Build history of the part. All positions in model axes, mm. A direction names the side the tool comes from. Round coordinates to 2 decimals unless told otherwise and drop trailing zeros. Write each loop counter-clockwise with the first axis right and the second up, starting at its lowest first coordinate (ties: lowest second). Pieces come first, ordered by that corner, then holes.
Item 1: Wall check: probe 1 along Y at (x, z) = (-3, 3.65); probe 2 along X at (y, z) = (5, 0.25); probe 3 along Y at (x, z) = (-14, 3.25). Give the ranges that are in metal, low to high.
Item 2: Band-saw the part on B-B, the plane y = 4.5. Write the cut outline in (x, z), then the cut area to 4 significant figures.
Item 3: Band-saw the part on A-A, the plane x = 3. Write the cut outline in (y, z).
Item 4: 3-axis set-ups, long thin cutter, end or side, ignore diameter. For faces 5 (the flat face through (-16, -6.3, 2)), 6 (the flat face through (-6.2, -9, 2)), 7 (the flat face through (-15.25, 4.6, 2.5)), 8 (the flat face through (16, 4.1, 2)): which of +Z, -Z, +X, -X, +Y, -Y reach the whole face in a straight line?
Item 5: Drop flat-ended pins along their axis: pin 1 Ø1.5 at (y, z) = (-4, 1.5) entering from +X; pin 2 Ø1 at (x, z) = (-16, 1.5) entering from +Y; pin 3 Ø0.5 at (y, z) = (6.5, 3.5) entering from -X. Give the stop position or say it passes through.
Item 6: Mould opens along X. For faces 1 (the flat face through (-16, 4.1, 2)), 2 (the flat face through (-5.946, -6.838, 2.465)), 3 (the flat face through (8.6, 6.5, 2.5)), 4 (the flat face through (-16.45, -7, 2)) say: +X half, -X half, draft (parallel to the pull), parting line (faces both ways), or undercut.
```python
from build123d import *

# Parameters (mm, degrees)
COMPONENT_OUTLINE_DEPTH = 5


with BuildPart() as part:
    # 草图1 → Component_Outline (new body)
    with BuildSketch(Plane.XY):
        Polygon((-13.6, -10.7), (-13.6, -7.7), (-16.45, -7.7), (-16.45, -6.3), (-15.5, -6.3), (-15.2844, -6.2894), (-15.0708, -6.2577), (-14.8614, -6.2053), (-14.6581, -6.1325), (-14.4629, -6.0402), (-14.2778, -5.9292), (-14.1043, -5.8006), (-13.9444, -5.6556), (-13.7994, -5.4957), (-13.6708, -5.3223), (-13.5598, -5.1371), (-13.4675, -4.9419), (-13.3947, -4.7386), (-13.3423, -4.5292), (-13.3106, -4.3157), (-13.3, -4.1), (-13.3106, -3.8844), (-13.3423, -3.6708), (-13.3947, -3.4614), (-13.4675, -3.2581), (-13.5598, -3.0629), (-13.6708, -2.8777), (-13.7994, -2.7043), (-13.9444, -2.5444), (-14.1043, -2.3994), (-14.2778, -2.2708), (-14.4629, -2.1598), (-14.6581, -2.0675), (-14.8614, -1.9947), (-15.0708, -1.9423), (-15.2844, -1.9106), (-15.5, -1.9), (-16.45, -1.9), (-16.45, 4.1), (-15.25, 4.1), (-15.25, 5.1), (-9.3, 5.85), (-6, 6.05), (-6, 7.1), (8.6, 7.1), (8.6, 5.9), (9.3, 5.85), (15.25, 5.1), (15.25, 4.1), (16.45, 4.1), (16.45, -1.9), (15.5, -1.9), (15.2844, -1.9106), (15.0708, -1.9423), (14.8614, -1.9947), (14.6581, -2.0675), (14.4629, -2.1598), (14.2778, -2.2708), (14.1043, -2.3994), (13.9444, -2.5444), (13.7994, -2.7043), (13.6708, -2.8777), (13.5598, -3.0629), (13.4675, -3.2581), (13.3947, -3.4614), (13.3423, -3.6708), (13.3106, -3.8844), (13.3, -4.1), (13.3106, -4.3157), (13.3423, -4.5292), (13.3947, -4.7386), (13.4675, -4.9419), (13.5598, -5.1371), (13.6708, -5.3223), (13.7994, -5.4957), (13.9444, -5.6556), (14.1043, -5.8006), (14.2778, -5.9292), (14.4629, -6.0402), (14.6581, -6.1325), (14.8614, -6.2053), (15.0708, -6.2577), (15.2844, -6.2894), (15.5, -6.3), (16.45, -6.3), (16.45, -7.7), (13.3, -7.7), (12.15, -6), (-5.7, -6), (-6.2, -7.7), (-6.2, -10.7), align=None)
    extrude(amount=COMPONENT_OUTLINE_DEPTH)


solid = part.part
```
Results:
1. probe 1: y = -6 to 7.1
1. probe 2: x = -15.25 to 15.25
1. probe 3: y = -7.7 to -5.71, -2.49 to 5.26
2. outline: (-15.25, 0) - (15.25, 0) - (15.25, 5) - (-15.25, 5) - close
2. area: 152.5 mm2
3. outline: (-6, 0) - (7.1, 0) - (7.1, 5) - (-6, 5) - close
4. face 5: +Z, -Z, -X
4. face 6: +Z, -Z, +X, -Y
4. face 7: +Z, -Z, -X, +Y
4. face 8: +Z, -Z, +X, +Y
5. pin 1: stops at x = 13.47
5. pin 2: stops at y = 4.1
5. pin 3: stops at x = -6
6. face 1: draft
6. face 2: undercut
6. face 3: +X half
6. face 4: -X half
